```python
from build123d import *

# Parameters (mm, degrees)
SALIENTE_EXTRUIR1_DEPTH = 7.5
CROQUIS3_R              = 3
CORTAR_EXTRUIR1_DEPTH   = 57.124860802


with BuildPart() as part:
    # Croquis2 → Saliente-Extruir1 (new, symmetric)
    with BuildSketch(Plane.XY):
        with BuildLine():
            Line((0, 0), (-30, 0))
            Line((-30, 0), (-30, 30))
            ThreePointArc((-30, 30), (-15, 45), (0, 30))
            Line((0, 30), (0, 0))
        make_face()
    extrude(amount=SALIENTE_EXTRUIR1_DEPTH, both=True)

    # Croquis3 → Cortar-Extruir1 (cut, through all)
    with BuildSketch(Plane.XY.offset(7.5)):
        with Locations((-15, 30)):
            Circle(CROQUIS3_R)
    extrude(amount=-CORTAR_EXTRUIR1_DEPTH, mode=Mode.SUBTRACT)


solid = part.part
```
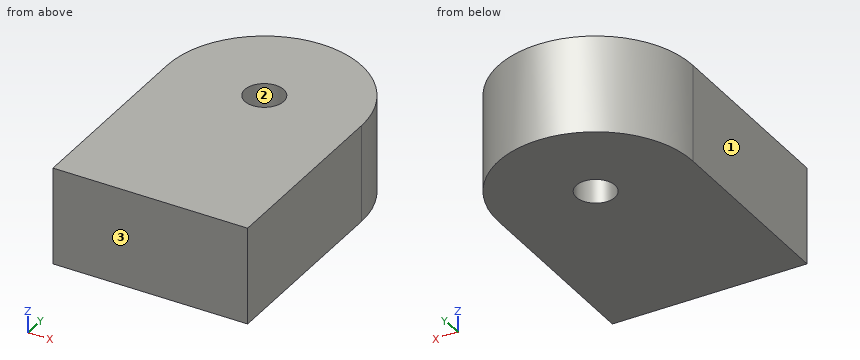
Geometry check sheet. Reference: the model listing, model coordinates, mm. Face numbers are marked on the shaded views. Round coordinates to 2 decimals unless told otherwise and drop trailing zeros. Loops run counter-clockwise (first coordinate to the right, second up) from the corner with the lowest first, then second, coordinate; pieces in that order, holes last. Notation, with made-up numbers: (38, 66) - (96, 66) arc R9 ccw to (96, 81) - close; hole circle Ø8 at (45, 19). An arc over 180 degrees is marked (long way). Write item = value, one per line. Start each with the question number.
1. Section check D-D on x = -3.5. Enter the section's corners in (y, z), then the cut area to 3 significant figures.
2. Section check B-B on y = 30.5. Enter the section's corners in (x, z), then the cut area to 3 significant figures.
3. Thickness scan on line 1 (Y direction, x = -15, z = -3.25); line 2 (X direction, y = 42, z = -5); line 3 (Y direction, x = -2.5, z = 0). Record the ranges inside material, lowest first.
4. Section check C-C on z = -1.5. Enter the section's corners in (x, y), then the cut area to 3 significant figures.
5. Mould release check, pull along Y, two halves, no side actions. Record for the marked faces 1, 2 and 3: released by +Y, released by -Y, zero draft, split by the parting line, or undercut.
6. Depth check by flat-ended pin: pin 1 (5 mm diameter, centred on x = -10, z = 4, fed in from +Y); pin 2 (1 mm diameter, centred on x = -23.5, z = -2.5, fed in from +Y); pin 3 (4 mm diameter, centred on x = -23, z = 4, fed in from +Y). Enter the tip coordinate at first touch or a pass-through.
7. Section check A-A on x = -15. Enter the section's corners in (y, z).
Working result:
q1.outline = (0, -7.5) - (39.63, -7.5) - (39.63, 7.5) - (0, 7.5) - close
q1.area = 594 mm^2
q2.outline = (-29.99, -7.5) - (-17.96, -7.5) - (-17.96, 7.5) - (-29.99, 7.5) - close; (-12.04, -7.5) - (-0.01, -7.5) - (-0.01, 7.5) - (-12.04, 7.5) - close
q2.area = 361 mm^2
q3.line_1 = 0 to 27, 33 to 45
q3.line_2 = -24 to -6
q3.line_3 = 0 to 38.29
q4.outline = (-30, 0) - (0, 0) - (0, 30) arc R15 ccw to (-30, 30) - close; hole circle Ø6 at (-15, 30)
q4.area = 1,230 mm^2
q5.face_1 = zero draft
q5.face_2 = undercut
q5.face_3 = released by -Y
q6.pin_1 = 44.79
q6.pin_2 = 42.69
q6.pin_3 = 43.75
q7.outline = (0, -7.5) - (27, -7.5) - (27, 7.5) - (0, 7.5) - close; (33, -7.5) - (45, -7.5) - (45, 7.5) - (33, 7.5) - close
